Check sheet for the modelled part. Datum: model origin and axes. Units: mm. A direction names the side the tool comes from. Give positions to 0.01 mm unless a question says otherwise; leave off trailing zeros. Order: outer loops, then holes, each group sorted by start corner. A loop starts at its lowest first (then second) coordinate and runs counter-clockwise, first axis right, second up.
```python
from build123d import *

# Parameters (mm, degrees)
SKETCH1_W       = 3
SKETCH1_H       = 2.5
EXTRUDE1_DEPTH  = 4
SKETCH2_W       = 0.645
SKETCH2_H       = 6
EXTRUDE2_DEPTH  = 0.64
LPATTERN1_COUNT = 3
LPATTERN1_PITCH = 2.54
CHAMFER1_SIZE   = 0.25


with BuildPart() as part:
    # Sketch1 → Extrude1 (new body, symmetric)
    with BuildSketch(Plane.XY):
        Rectangle(SKETCH1_W, SKETCH1_H)
    extrude(amount=EXTRUDE1_DEPTH, both=True)

    # Sketch2 → Extrude2 (add)
    with BuildSketch(Plane.XY.offset(2.86)):
        with BuildLine():
            Line((-0.3225, 1.25), (-0.3225, 2.245))
            ThreePointArc((-0.3225, 2.245), (-0.374776878, 2.375), (-0.5025, 2.43261663))
            Line((-0.5025, 2.43261663), (-4.0025, 2.43261663))
            Line((-4.0025, 2.43261663), (-4.0025, 3.06831282))
            Line((-4.0025, 3.06831282), (-0.4975, 3.06831282))
            ThreePointArc((-0.4975, 3.06831282), (0.082527742, 2.826), (0.3225, 2.245))
            Line((0.3225, 2.245), (0.3225, 1.25))
            Line((0.3225, 1.25), (-0.3225, 1.25))
        make_face()
        with Locations((0, -4.25)):
            Rectangle(SKETCH2_W, SKETCH2_H)
    extrude2 = extrude(amount=-EXTRUDE2_DEPTH)

    # LPattern1: Extrude2 ×3
    with Locations(*[(0, 0, -i * LPATTERN1_PITCH) for i in range(1, LPATTERN1_COUNT)]):
        add(extrude2)

    # Chamfer1
    chamfer1_edges = [part.edges().sort_by_distance(p)[0] for p in [
        (-4.0025, 2.750464725, 2.22),
        (-4.0025, 2.43261663, 2.54),
        (-4.0025, 3.06831282, 2.54),
        (-4.0025, 2.750464725, 2.86),
        (0, -7.25, 2.22),
        (0.3225, -7.25, 2.54),
        (-0.3225, -7.25, 2.54),
        (0, -7.25, 2.86),
        (-4.0025, 2.750464725, -0.32),
        (-4.0025, 2.43261663, 0),
        (-4.0025, 3.06831282, 0),
        (-4.0025, 2.750464725, 0.32),
        (0, -7.25, -0.32),
        (0.3225, -7.25, 0),
        (-0.3225, -7.25, 0),
        (0, -7.25, 0.32),
        (-4.0025, 2.750464725, -2.86),
        (-4.0025, 2.43261663, -2.54),
        (-4.0025, 3.06831282, -2.54),
        (-4.0025, 2.750464725, -2.22),
        (0, -7.25, -2.86),
        (0.3225, -7.25, -2.54),
        (-0.3225, -7.25, -2.54),
        (0, -7.25, -2.22),
    ]]
    chamfer(chamfer1_edges, length=CHAMFER1_SIZE)


solid = part.part
```
(1) Gauge pin test, flat ends, axial feed: pin 1 Ø0.5 at (x, y) = (0, -5) entering from +Z; pin 2 Ø0.7 at (y, z) = (-4, 2.5) entering from -X; pin 3 Ø3 at (y, z) = (-6, 0) entering from +X. Record the tip position at first contact, or that the pin passes through.
Response values:
pin 1: stops at z = 2.86
pin 2: stops at x = -0.32
pin 3: stops at x = 0.32
(2) Cross-section at C-C on x = -1.05. Enter the section's corners in (y, z).
Response values:
outline: (-1.25, -4) - (1.25, -4) - (1.25, 4) - (-1.25, 4) - close; (2.43, -2.86) - (3.07, -2.86) - (3.07, -2.22) - (2.43, -2.22) - close; (2.43, -0.32) - (3.07, -0.32) - (3.07, 0.32) - (2.43, 0.32) - close; (2.43, 2.22) - (3.07, 2.22) - (3.07, 2.86) - (2.43, 2.86) - close
(3) Cross-section at D-D on z = 1.5. Enter the section's corners in (x, y), then the cut area to 3 significant figures.
Response values:
outline: (-1.5, -1.25) - (1.5, -1.25) - (1.5, 1.25) - (-1.5, 1.25) - close
area: 7.50 mm2
(4) Set-up check for faces 4 (the face through (-1, 1.25, 0)), 5 (the face through (-1.2, 2.6, 0.32)), 6 (the face through (0.08, 2.83, 2.54)), 7 (the face through (-1.2, 2.6, -2.86)), 8 (the face through (-1.5, 0, 0)): record each of +Z, -Z, +X, -X, +Y, -Y from which the full face is reachable in a straight line by a thin tool's end or side.
Response values:
face 4: none
face 5: +X, -X, +Y
face 6: +Z, -Z, +X, +Y
face 7: -Z, +X, -X, +Y
face 8: +Z, -Z, -X, -Y
(5) Material ranges on L1, parallel to X at y = -1, z = 1; L2, parallel to Y at x = 1.2, z = -2.5; L3, parallel to X at y = -3.25, z = 2.75, recorded low to high.
Response values:
L1: x = -1.5 to 1.5
L2: y = -1.25 to 1.25
L3: x = -0.32 to 0.32
(6) Cross-section at B-B on y = -3.75. Enter the section's corners in (x, z), then the cut area to 3 significant figures.
Response values:
outline: (-0.32, -2.86) - (0.32, -2.86) - (0.32, -2.22) - (-0.32, -2.22) - close; (-0.32, -0.32) - (0.32, -0.32) - (0.32, 0.32) - (-0.32, 0.32) - close; (-0.32, 2.22) - (0.32, 2.22) - (0.32, 2.86) - (-0.32, 2.86) - close
area: 1.24 mm2
(7) Cross-section at A-A on x = -1.9. Enter the section's corners in (y, z), then the cut area to 3 significant figures.
Response values:
outline: (2.43, -2.86) - (3.07, -2.86) - (3.07, -2.22) - (2.43, -2.22) - close; (2.43, -0.32) - (3.07, -0.32) - (3.07, 0.32) - (2.43, 0.32) - close; (2.43, 2.22) - (3.07, 2.22) - (3.07, 2.86) - (2.43, 2.86) - close
area: 1.22 mm2
(8) Release check for a two-part mould opening along Z. For faces 1 (the face through (-1.2, 2.6, 2.86)), 2 (the face through (-1.2, 2.6, 2.22)), 3 (the face through (0.08, 2.83, -2.54)) record: released by +Z, released by -Z, zero draft, split by the parting line, or undercut.
Response values:
face 1: released by +Z
face 2: undercut
face 3: zero draft
